Geometry: final body of the model. Coordinates: model frame, mm. A direction names the side the tool comes from. Give positions to 0.01 mm unless a question says otherwise; leave off trailing zeros. Write each loop counter-clockwise with the first axis right and the second up, starting at its lowest first coordinate (ties: lowest second). Pieces come first, ordered by that corner, then holes.
from build123d import *

# Parameters (mm, degrees)
F0_W     = 19.05
F0_H     = 19.05
F0_R     = 4.7625
F1_DEPTH = 7.9375
F2_R     = 3.175
F3_R     = 1.35255
F4_DEPTH = 4.7625
F5_R     = 1.7272
F6_DEPTH = 6.0867362041


with BuildPart() as f1:
    # F0 (on Top) → F1 (new body)
    with BuildSketch(Plane.XY):
        Rectangle(F0_W, F0_H)
        Circle(F0_R, mode=Mode.SUBTRACT)
    extrude(amount=F1_DEPTH)

    # F2
    f2_edges = [f1.edges().sort_by_distance(p)[0] for p in [
        (-9.525, 9.525, 3.96875),
        (-9.525, -9.525, 3.96875),
        (9.525, -9.525, 3.96875),
        (9.525, 9.525, 3.96875),
    ]]
    fillet(f2_edges, radius=F2_R)

    # F3 (on face) → F4 (cut)
    with BuildSketch(Plane(origin=(0, 0, 0), x_dir=(1, 0, 0), z_dir=(0, 0, -1))):
        with Locations((6.35, 6.35)):
            Circle(F3_R)
        with Locations((-6.35, 6.35)):
            Circle(F3_R)
        with Locations((-6.35, -6.35)):
            Circle(F3_R)
        with Locations((6.35, -6.35)):
            Circle(F3_R)
    extrude(amount=-F4_DEPTH, mode=Mode.SUBTRACT)

    # F5 (on face) → F6 (cut, up to face)
    with BuildSketch(Plane.YZ.offset(9.525)):
        with Locations((0, 3.96875)):
            Circle(F5_R)
    extrude(amount=-F6_DEPTH, mode=Mode.SUBTRACT)


solid = f1.part
Q1. Ray query, line 1 along Y through (x, z) = (-6.35, 1) (3 decimals); line 2 along Z through (x, y) = (5.7, 0). Return the intervals inside material, ascending.
Filled sheet:
line 1: y = -9.525 to -7.703, -4.997 to 4.997, 7.703 to 9.525
line 2: z = 0 to 2.24, 5.7 to 7.94
Q2. Section D-D on y = 0.25. Output: boundary loops of the cut face in (x, z) (1 decimal), plus the area to 3 significant figures.
Filled sheet:
outline: (-9.5, 0) - (-4.8, 0) - (-4.8, 7.9) - (-9.5, 7.9) - close; (4.8, 0) - (9.5, 0) - (9.5, 2.3) - (4.8, 2.3) - close; (4.8, 5.7) - (9.5, 5.7) - (9.5, 7.9) - (4.8, 7.9) - close
area: 59.4 mm2
Q3. Pull-direction query (Y, two-part tool) for faces 4 (the flat face through (-2.3, 4.4, 0)), 5 (the flat face through (-6, -6, 4.762)), 6 (the cylindrical face through (8.57, 8.62, 4.02)), 7 (the flat face through (6, 6, 4.762)); classes: released by +Y, released by -Y, zero draft, split by the parting line, or undercut.
Filled sheet:
face 4: zero draft
face 5: undercut
face 6: released by +Y
face 7: undercut
Q4. Section A-A on x = 0. Output: boundary loops of the cut face in (y, z) (1 decimal).
Filled sheet:
outline: (-9.5, 0) - (-4.8, 0) - (-4.8, 7.9) - (-9.5, 7.9) - close; (4.8, 0) - (9.5, 0) - (9.5, 7.9) - (4.8, 7.9) - close
Q5. Pin query (flat end, axial travel): P1, Ø2, axis at x = 6.35, y = 6.35, coming from the -Z side; P2, Ø5.5, axis at x = 0, y = 0, coming from the +Z side; P3, Ø2, axis at y = 7.5, z = 3.5, coming from the +X side; P4, Ø2, axis at x = 7.5, z = 2, coming from the +Y side. Return the tip coordinate at first contact, or that it passes through.
Filled sheet:
P1: stops at z = 4.76
P2: passes through
P3: stops at x = 9.52
P4: stops at y = 9.52
Q6. Access query for faces 1 (the cylindrical face through (7.02, -0.37, 2.28)), 2 (the cylindrical face through (-7.4, 7.2, 2.3)), 3 (the flat face through (-9.525, 0, 4)). Directions: +Z, -Z, +X, -X, +Y, -Y. A direction counts if a zero-diameter tool reaches every point of the face in a straight line with its end or side. Return the directions, or none.
Filled sheet:
face 1: +X
face 2: -Z
face 3: +Z, -Z, -X, +Y, -Y
Q7. Section C-C on y = -4.5. Output: boundary loops of the cut face in (x, z) (1 decimal), plus the area to 3 significant figures.
Filled sheet:
outline: (-9.5, 0) - (-1.6, 0) - (-1.6, 7.9) - (-9.5, 7.9) - close; (1.6, 0) - (9.5, 0) - (9.5, 7.9) - (1.6, 7.9) - close
area: 126 mm2
